Here's how the part is built. I have some questions about the finished solid (model axes, mm). A direction names the side the tool comes from. Coordinates: 2 decimals unless noted, no trailing zeros. Write each loop counter-clockwise with the first axis right and the second up, starting at its lowest first coordinate (ties: lowest second). Pieces come first, ordered by that corner, then holes. Notation, with made-up numbers: (54.25, 62) -> (80.25, 62) arc R21 ccw to (80.25, 67) -> close; hole circle Ø1 at (7, 60.5). An arc over 180 degrees is marked (long way). Use a Markdown table: item, result. Add a question column.
Item 1: Imagine slicing it at C-C, the plane y = 5.5. Write out the boundary of the cut face in (x, z), and give its area (3 significant figures).
Item 2: Imagine slicing it at A-A, the plane y = -10. Write out the boundary of the cut face in (x, z).
Item 3: If we mould it in two halves opening along X, with no side actions, what happens to faces 1 (the flat face through (21, -1, 0)), 2 (the cylindrical face through (23.028, 11.486, 19.297)), 3 (the cylindrical face through (9.55, -15.53, -12.3)), 4 (the flat face through (25, -4, 0))? For each: pulls with the +X half, pulls with the -X half, needs draft (parallel to the pull), parting line crosses it, or undercut.
Item 4: If I drill on line 1 along Z through (x, y) = (12.5, -15.3); line 2 along X through (y, z) = (-8.5, -19); line 3 along Y through (x, z) = (12.5, 5), over which ranges is the centre line in solid material (lowest first)? Write a range as from..to.
Item 5: Imagine slicing it at D-D, the plane z = -14. Write out the boundary of the cut face in (x, y).
Item 6: On a 3-axis mill with a long thin cutter (end or side, diameter ignored), from which of +Z, -Z, +X, -X, +Y, -Y can I reach the whole of each face in a straight line? I mean faces 5 (the flat face through (12, -17.5, 0)), 6 (the flat face through (12, -13.5, 0)). Say none if no direction works.
Item 7: Imagine slicing it at B-B, the plane z = 0. Write out the boundary of the cut face in (x, y).
```python
from build123d import *

# Parameters (mm, degrees)
SKETCH1_W           = 50
SKETCH1_H           = 35
BOSS_EXTRUDE1_DEPTH = 25
SKETCH2_W           = 17
SKETCH2_H           = 50
CUT_EXTRUDE1_DEPTH  = 31
SKETCH4_R           = 6
CUT_EXTRUDE2_DEPTH  = 26
SKETCH5_R           = 4
CUT_EXTRUDE3_DEPTH  = 4
FILLET1_R           = 20


with BuildPart() as part:
    # Sketch1 → Boss-Extrude1 (new body)
    with BuildSketch(Plane(origin=(0, 0, 0), x_dir=(0, 0, -1), z_dir=(1, 0, 0))):
        Rectangle(SKETCH1_W, SKETCH1_H)
    extrude(amount=BOSS_EXTRUDE1_DEPTH)

    # Sketch2 → Cut-Extrude1 (cut)
    with BuildSketch(Plane(origin=(0, 17.5, 0), x_dir=(1, 0, 0), z_dir=(0, 1, 0))):
        with Locations((12.5, 0)):
            Rectangle(SKETCH2_W, SKETCH2_H)
    extrude(amount=-CUT_EXTRUDE1_DEPTH, mode=Mode.SUBTRACT)

    # Sketch4 → Cut-Extrude2 (cut, through all)
    with BuildSketch(Plane.ZY):
        with Locations((0, 5.5)):
            Circle(SKETCH4_R)
    extrude(amount=-CUT_EXTRUDE2_DEPTH, mode=Mode.SUBTRACT)

    # Sketch5 → Cut-Extrude3 (cut)
    with BuildSketch(Plane.XZ.offset(17.5)):
        with Locations((12.5, 15)):
            Circle(SKETCH5_R)
        with Locations((12.5, -15)):
            Circle(SKETCH5_R)
    extrude(amount=-CUT_EXTRUDE3_DEPTH, mode=Mode.SUBTRACT)

    # Fillet1
    fillet1_edges = [part.edges().sort_by_distance(p)[0] for p in [
        (2, 17.5, 25),
        (2, 17.5, -25),
        (23, 17.5, 25),
        (23, 17.5, -25),
    ]]
    fillet(fillet1_edges, radius=FILLET1_R)


solid = part.part
```
Ans:
| question | item | result |
|---|---|---|
| 1 | outline | (0, -23.33) -> (4, -23.33) -> (4, -6) -> (0, -6) -> close; (0, 6) -> (4, 6) -> (4, 23.33) -> (0, 23.33) -> close; (21, -23.33) -> (25, -23.33) -> (25, -6) -> (21, -6) -> close; (21, 6) -> (25, 6) -> (25, 23.33) -> (21, 23.33) -> close |
| 1 | area | 277 mm^2 |
| 2 | outline | (0, -25) -> (4, -25) -> (4, 25) -> (0, 25) -> close; (21, -25) -> (25, -25) -> (25, 25) -> (21, 25) -> close |
| 3 | face 1 | undercut |
| 3 | face 2 | needs draft |
| 3 | face 3 | undercut |
| 3 | face 4 | pulls with the +X half |
| 4 | line 1 | z = -25..-19, -11..11, 19..25 |
| 4 | line 2 | x = 0..4, 21..25 |
| 4 | line 3 | y = -17.5..-13.5 |
| 5 | outline | (0, -17.5) -> (8.63, -17.5) -> (8.63, -13.5) -> (4, -13.5) -> (4, 15.36) -> (0, 15.36) -> close; (16.37, -17.5) -> (25, -17.5) -> (25, 15.36) -> (21, 15.36) -> (21, -13.5) -> (16.37, -13.5) -> close |
| 6 | face 5 | +Z, -Z, +X, -X, -Y |
| 6 | face 6 | +Z, -Z, +Y |
| 7 | outline | (0, -17.5) -> (25, -17.5) -> (25, -0.5) -> (21, -0.5) -> (21, -13.5) -> (4, -13.5) -> (4, -0.5) -> (0, -0.5) -> close; (0, 11.5) -> (4, 11.5) -> (4, 17.5) -> (0, 17.5) -> close; (21, 11.5) -> (25, 11.5) -> (25, 17.5) -> (21, 17.5) -> close |
